Job drawing, mm, ordinate dimensions from the low corner. One solid piece. A direction names the side the tool comes from. Round coordinates to 2 decimals unless told otherwise and drop trailing zeros. Order: outer loops, then holes, each group sorted by start corner. A loop starts at its lowest first (then second) coordinate and runs counter-clockwise, first axis right, second up. Notation, with made-up numbers: (4.25, -22) -> (29.25, -22) arc R27 cw to (29.25, 15) -> close; hole circle Ø8 at (-26, -19). An arc over 180 degrees is marked (long way). Return JSON: item names as keys, results as strings. Group by question number.
Q1. Cut at D-D (x = 32.5). Write the cut outline in (y, z), then the cut area to 3 significant figures.
Q2. Cut at A-A (z = 5.56). Write the cut outline in (x, y).
Q3. Probe line 1 along Y through (x, z) = (19, 29.5); line 2 along X through (y, z) = (4, 12); line 3 along Y through (x, z) = (19, 29). List the from-to ranges inside material, lowest first.
Q4. Which spindle directions (+Z, -Z, +X, -X, +Y, -Y) get a long thin tool onto all of the face, cutting with end or side? Do the marked faces 4 and 5. Say none if no direction does.
Q5. Flat gauge pins, fed straight in: pin 1 (8 mm diameter, centred on x = 20.5, z = 28.5, fed in from +Y); pin 2 (2 mm diameter, centred on x = 12.5, z = 33.5, fed in from +Y); pin 3 (3 mm diameter, centred on x = 23, y = 29, fed in from +Z). Where does each tip first touch, or does it go through?
Q6. Mould opens along Z. For the marked faces 1, 2 and 3 say: +Z half, -Z half, draft (parallel to the pull), parting line (faces both ways), or undercut.
Q7. Cut at C-C (x = 14). Write the cut outline in (y, z) (1 decimal), then the cut area to 3 significant figures.
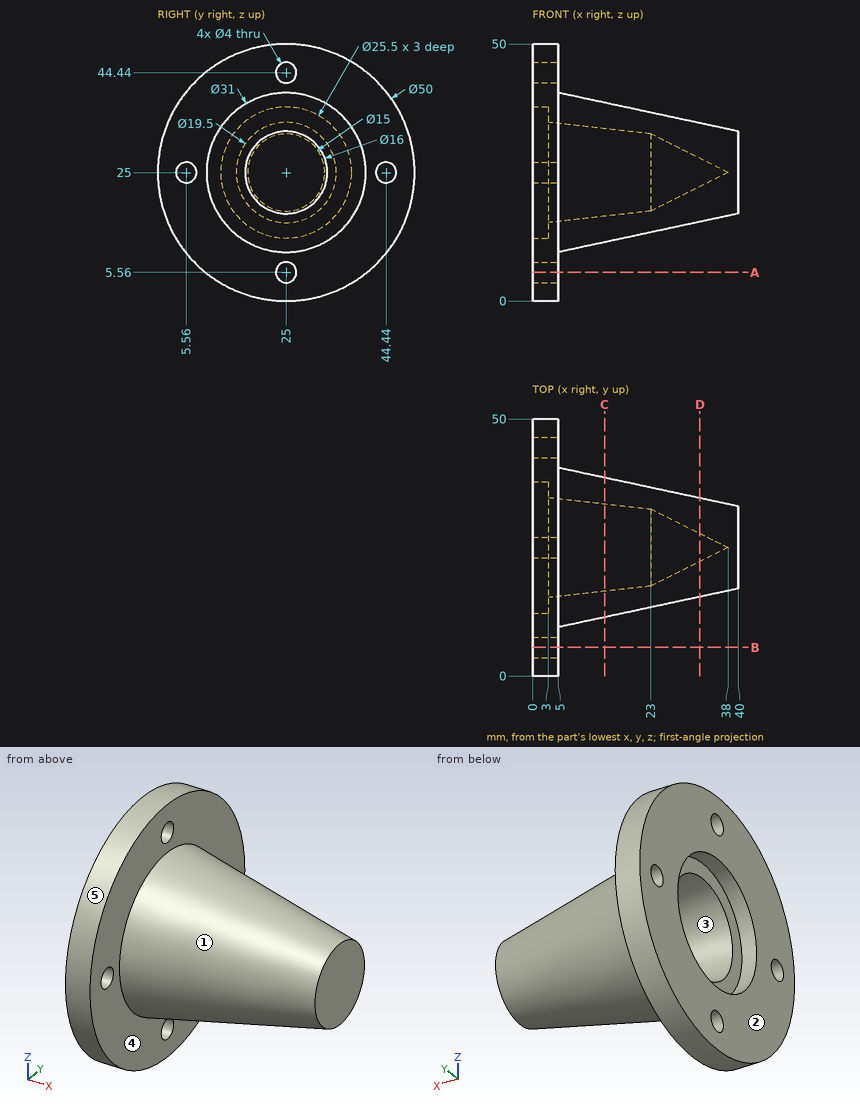
Solution:
{
 "1": {"outline": "circle Ø19.21 at (25, 25); hole circle Ø5.5 at (25, 25)", "area": "266 mm²"},
 "2": {"outline": "(0, 9.28) -> (5, 9.28) -> (5, 23) -> (0, 23) -> close; (0, 27) -> (5, 27) -> (5, 40.72) -> (0, 40.72) -> close"},
 "3": {"line 1": "y = 13.34 to 18.45, 31.55 to 36.66", "line 2": "x = 0 to 5", "line 3": "y = 13.16 to 18.13, 31.87 to 36.84"},
 "4": {"face 4": "+X", "face 5": "+X, -X"},
 "5": {"pin 1": "stops at y = 37.83", "pin 2": "stops at y = 36.74", "pin 3": "stops at z = 36.5"},
 "6": {"face 1": "parting line", "face 2": "draft", "face 3": "undercut"},
 "7": {"outline": "circle Ø27.1 at (25, 25); hole circle Ø17 at (25, 25)", "area": "351 mm²"}
}
